Here's how the part is built. I have some questions about the finished solid (model axes, mm). Round coordinates to 2 decimals unless told otherwise and drop trailing zeros. Order: outer loops, then holes, each group sorted by start corner. A loop starts at its lowest first (then second) coordinate and runs counter-clockwise, first axis right, second up. Notation, with made-up numbers: (-7, -27.75) -> (18, -27.75) arc R25 cw to (18, -7.75) -> close; hole circle Ø5 at (17, 70). An arc over 180 degrees is marked (long way). Use a Markdown table: item, result. Add a question column.
Autodesk Inventor part; units mm, degrees
ref_plane "YZ Plane" through (0, 0, 0) normal (1, 0, 0) x (0, 1, 0)
ref_plane "XZ Plane" through (0, 0, 0) normal (0, 1, 0) x (-1, 0, 0)
ref_plane "XY Plane" through (0, 0, 0) normal (0, 0, 1) x (1, 0, 0)
sketch "Esboço1" plane through (0, 0, 0) normal (0, 1, 0) x (-1, 0, 0)
  line L0 (149, 5) -> (-149, 5)
  line L1 (-149, 5) -> (-149, -5)
  line L2 (-149, -5) -> (149, -5)
  line L3 (149, -5) -> (149, 5)
  line L4 (149, 5) -> (-149, -5) construction
  line L5 (-149, 5) -> (149, -5) construction
  point P0 (0, 0)
  dimension "d0" = 298
  dimension "d1" = 10
extrude "Placa1" add sketch "Esboço1" along normal blind 0.5
sketch "Esboço2" plane through (0, 0, 0) normal (0, -1, 0) x (1, 0, 0)
  line L0 (149, -5) -> (-149, -5)
  line L1 (149, 5) -> (149, -5)
  line L2 (-149, -5) -> (-149, 5)
  point P0 (0, 0)
  point P1 (-99, -1)
  point P2 (99, -1)
  dimension "d3" = 4
  dimension "d4" = 4
  dimension "d5" = 50
  dimension "d6" = 50
hole "Furo1" at (-99, 0, -1) at (99, 0, -1) direction (0, 1, 0) diameter 3 end through all
equation "\"d12\" = Espessura"
equation "\"d2\" = Espessura"
equation "\"Raio_vergadura\" = Espessura"
equation "\"Largura_alívio_de_vergadura\" = Espessura"
equation "\"Profundidade_alívio_de_vergadura\" = 0.5 * Espessura"
equation "\"Tamanho_alívio_de_dobra\" = 4 * Espessura"
equation "\"Remanescente_mínimo\" = 2 * Espessura"
equation "\"Raiodetransição\" = Raio_vergadura"
equation "\"Tamanho_de_raio_de_Jacobi\" = Raio_vergadura"
equation "\"TamanhoFolga\" = Espessura"
properties part number "Lateral 1 Gaveta" material "PMMA plástico"
(1) Please list where these lines run through material, in increasing order: probe 1 along X at (y, z) = (0.35, -1); probe 2 along Z at (x, y) = (99, 0.3); probe 3 along Z at (x, y) = (98, 0.2). Write a range as from..to.
(2) I want a section at A-A on z = -1. List the corners of the cut face in (x, y) for me, and give its area (3 significant figures).
(3) I'm going to push a flat-ended pin straight in: P1, Ø2.5, axis at x = -99, z = -1, coming from the -Y side. Where does the tip first touch, or does it pass through?
Output:
| question | item | result |
|---|---|---|
| 1 | probe 1 | -149..-100.5, -97.5..97.5, 100.5..149 |
| 1 | probe 2 | -5..-2.5, 0.5..5 |
| 1 | probe 3 | -5..-2.12, 0.12..5 |
| 2 | outline | (-149, 0) -> (-100.5, 0) -> (-100.5, 0.5) -> (-149, 0.5) -> close; (-97.5, 0) -> (97.5, 0) -> (97.5, 0.5) -> (-97.5, 0.5) -> close; (100.5, 0) -> (149, 0) -> (149, 0.5) -> (100.5, 0.5) -> close |
| 2 | area | 146 mm² |
| 3 | P1 | through |
